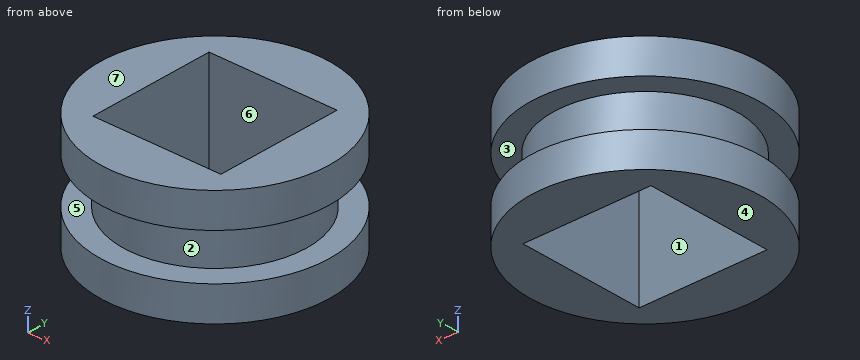
```python
from build123d import *

# Parameters (mm, degrees)
F2_W     = 7.112
F2_H     = 7.112
F3_DEPTH = 25.4


with BuildPart() as f1:
    # F0 (on Front) → F1 (revolve)
    with BuildSketch(Plane.XZ):
        Polygon((0, 6.35), (0, 0), (6.35, 0), (6.35, 1.905), (5.08, 1.905), (5.08, 4.445), (6.35, 4.445), (6.35, 6.35), align=None)
    revolve(axis=Axis((0, 0, 3.175), (0, 0, 1)))

    # F2 (on face) → F3 (cut)
    with BuildSketch(Plane(origin=(0, 0, 0), x_dir=(1, 0, 0), z_dir=(0, 0, -1))):
        Rectangle(F2_W, F2_H)
    extrude(amount=-F3_DEPTH, mode=Mode.SUBTRACT)


solid = f1.part
```
The model under review builds one solid part; all positions refer to its coordinate system, in mm. Face numbers are marked on the shaded views. A direction names the side the tool comes from. Round coordinates to 2 decimals unless told otherwise and drop trailing zeros. Write each loop counter-clockwise with the first axis right and the second up, starting at its lowest first coordinate (ties: lowest second). Pieces come first, ordered by that corner, then holes.
(1) Machinability: for the marked faces 5, 6 and 7, which of the approach directions +Z, -Z, +X, -X, +Y, -Y give a long, thin tool a straight path to every point of the face, cutting with its end or side? Answer none if there is none.
(2) We need section B-B on x = 0.75. Give the boundary of the cut face in (y, z) (3 decimals).
(3) We need section A-A on y = 0. Give the boundary of the cut face in (x, z) (3 decimals).
(4) Insertion check: pin 1 (1.9 mm diameter, centred on y = 1, z = 3, fed in from -X); pin 2 (3 mm diameter, centred on x = -4.5, z = 5, fed in from +Y); pin 3 (1.5 mm diameter, centred on y = 2.5, z = 5, fed in from +X). Each pin has a flat end and moves straight along its axis. Give the tip position at first contact, or say it passes through.
(5) Mouldability with a two-part tool opening along Z and no side actions: class the marked faces 1, 2, 3 and 4 as +Z half, -Z half, draft (parallel to the pull), parting line (faces both ways), or undercut.
(6) Wall thickness on L1, parallel to Z at x = -1.75, y = 5.5 (3 decimals); L2, parallel to Y at x = 1.25, z = 1; L3, parallel to Y at x = -2.75, z = 5: over which ranges is each line inside the solid? List them lowest first.
(7) We need section D-D on x = 5.25. Give the boundary of the cut face in (y, z) (3 decimals), and give its area (3 significant figures).
(8) We need section C-C on z = 0.75. Give the boundary of the cut face in (x, y), and give its area (3 significant figures).
Findings below:
1. face 5: none
1. face 6: +Z, -Z
1. face 7: +Z, +X, -X, +Y, -Y
2. outline: (-6.306, 0) - (-3.556, 0) - (-3.556, 6.35) - (-6.306, 6.35) - (-6.306, 4.445) - (-5.024, 4.445) - (-5.024, 1.905) - (-6.306, 1.905) - close; (3.556, 0) - (6.306, 0) - (6.306, 1.905) - (5.024, 1.905) - (5.024, 4.445) - (6.306, 4.445) - (6.306, 6.35) - (3.556, 6.35) - close
3. outline: (-6.35, 0) - (-3.556, 0) - (-3.556, 6.35) - (-6.35, 6.35) - (-6.35, 4.445) - (-5.08, 4.445) - (-5.08, 1.905) - (-6.35, 1.905) - close; (3.556, 0) - (6.35, 0) - (6.35, 1.905) - (5.08, 1.905) - (5.08, 4.445) - (6.35, 4.445) - (6.35, 6.35) - (3.556, 6.35) - close
4. pin 1: stops at x = -5.08
4. pin 2: stops at y = 5.6
4. pin 3: stops at x = 6.1
5. face 1: draft
5. face 2: undercut
5. face 3: undercut
5. face 4: -Z half
6. L1: z = 0 to 1.905, 4.445 to 6.35
6. L2: y = -6.23 to -3.56, 3.56 to 6.23
6. L3: y = -5.72 to -3.56, 3.56 to 5.72
7. outline: (-3.572, 0) - (3.572, 0) - (3.572, 1.905) - (-3.572, 1.905) - close; (-3.572, 4.445) - (3.572, 4.445) - (3.572, 6.35) - (-3.572, 6.35) - close
7. area: 27.2 mm2
8. outline: circle Ø12.7 at (0, 0); hole (-3.56, -3.56) - (3.56, -3.56) - (3.56, 3.56) - (-3.56, 3.56) - close
8. area: 76.1 mm2
